Design review of the part built by this model. Coordinates are the model's own, in mm. A direction names the side the tool comes from. Coordinates: 2 decimals unless noted, no trailing zeros. Loops run counter-clockwise (first coordinate to the right, second up) from the corner with the lowest first, then second, coordinate; pieces in that order, holes last. Notation, with made-up numbers: (-19.75, -27) -> (36.25, -27) arc R25 cw to (36.25, 5) -> close; hole circle Ø8 at (-35.5, 86.25). An arc over 180 degrees is marked (long way). Use CSV: the item, a comma, the result in double quotes.
```python
from build123d import *

# Parameters (mm, degrees)
AUFSATZ_LINEAR_AUSTRAGEN1_DEPTH        = 6
F_3_5_3_5_DURCHMESSER_BOHRUNG1_D       = 3.5
F_3_0_3_DURCHMESSER_BOHRUNG2_OUTLINE_R = 1.5
F_3_0_3_DURCHMESSER_BOHRUNG2_DEPTH     = 6
SKIZZE10_R                             = 2.5
AUFSATZ_LINEAR_AUSTRAGEN2_DEPTH        = 4


# Read off the part's stored shape, not the designer's step: Ø3.0 (3) Durchmesser Bohrung2
with BuildPart() as part:
    # Skizze1 → Aufsatz-Linear austragen1 (new body)
    with BuildSketch(Plane.XY):
        with BuildLine():
            Line((-551.752498469, 213.343199998), (-551.752498469, 212.343199998))
            Line((-551.752498469, 212.343199998), (-555.752498469, 212.343199998))
            ThreePointArc((-555.752498469, 212.343199998), (-559.752498469, 208.343199998), (-555.752498469, 204.343199998))
            Line((-555.752498469, 204.343199998), (-551.752498469, 204.343199998))
            Line((-551.752498469, 204.343199998), (-551.752498469, 196.343199998))
            Line((-551.752498469, 196.343199998), (-555.752498469, 196.343199998))
            ThreePointArc((-555.752498469, 196.343199998), (-559.752498469, 192.343199998), (-555.752498469, 188.343199998))
            Line((-555.752498469, 188.343199998), (-551.752498469, 188.343199998))
            Line((-551.752498469, 188.343199998), (-551.752498469, 187.343199998))
            Line((-551.752498469, 187.343199998), (-532.752498469, 187.343199998))
            Line((-532.752498469, 187.343199998), (-532.752498469, 193.634996066))
            Line((-532.752498469, 193.634996066), (-519.752498469, 193.634996066))
            Line((-519.752498469, 193.634996066), (-519.752498469, 187.343199998))
            Line((-519.752498469, 187.343199998), (-500.752498469, 187.343199998))
            Line((-500.752498469, 187.343199998), (-500.752498469, 188.343199998))
            Line((-500.752498469, 188.343199998), (-496.752498469, 188.343199998))
            ThreePointArc((-496.752498469, 188.343199998), (-492.752498469, 192.343199998), (-496.752498469, 196.343199998))
            Line((-496.752498469, 196.343199998), (-500.752498469, 196.343199998))
            Line((-500.752498469, 196.343199998), (-500.752498469, 204.343199998))
            Line((-500.752498469, 204.343199998), (-496.752498469, 204.343199998))
            ThreePointArc((-496.752498469, 204.343199998), (-492.752498469, 208.343199998), (-496.752498469, 212.343199998))
            Line((-496.752498469, 212.343199998), (-500.752498469, 212.343199998))
            Line((-500.752498469, 212.343199998), (-500.752498469, 213.343199998))
            Line((-500.752498469, 213.343199998), (-551.752498469, 213.343199998))
        make_face()
    extrude(amount=AUFSATZ_LINEAR_AUSTRAGEN1_DEPTH)

    # Ø3.5 (3.5) Durchmesser Bohrung1 (through all)
    with Locations(Plane.XY.offset(6)):
        with Locations((-555.752498469, 208.343199998), (-555.752498469, 192.343199998), (-496.752498469, 192.343199998), (-496.752498469, 208.343199998)):
            Hole(F_3_5_3_5_DURCHMESSER_BOHRUNG1_D / 2)

    # Ø3.0 (3) Durchmesser Bohrung2 outline → Ø3.0 (3) Durchmesser Bohrung2 (cut)
    with BuildSketch(Plane.XY):
        with Locations((-546.902498469, 208.493199998)):
            Circle(F_3_0_3_DURCHMESSER_BOHRUNG2_OUTLINE_R)
        with Locations((-505.602498469, 192.193199998)):
            Circle(F_3_0_3_DURCHMESSER_BOHRUNG2_OUTLINE_R)
        with Locations((-546.902498469, 192.193199998)):
            Circle(F_3_0_3_DURCHMESSER_BOHRUNG2_OUTLINE_R)
        with Locations((-505.602498469, 208.493199998)):
            Circle(F_3_0_3_DURCHMESSER_BOHRUNG2_OUTLINE_R)
    extrude(amount=F_3_0_3_DURCHMESSER_BOHRUNG2_DEPTH, mode=Mode.SUBTRACT)

    # Skizze10 → Aufsatz-Linear austragen2 (add)
    with BuildSketch(Plane.XY.offset(6)):
        with Locations((-546.902498469, 208.493199998)):
            Circle(SKIZZE10_R)
        with Locations((-546.902498469, 192.193199998)):
            Circle(SKIZZE10_R)
        with Locations((-505.602498469, 208.493199998)):
            Circle(SKIZZE10_R)
        with Locations((-505.602498469, 192.193199998)):
            Circle(SKIZZE10_R)
    extrude(amount=AUFSATZ_LINEAR_AUSTRAGEN2_DEPTH)


solid = part.part
```
Item 1: Add section D-D (z = 8.75). Give the boundary of the cut face in (x, y).
Checked values:
outline,"circle Ø5 at (-546.9, 192.19); circle Ø5 at (-546.9, 208.49); circle Ø5 at (-505.6, 192.19); circle Ø5 at (-505.6, 208.49)"
Item 2: Add section C-C (y = 202.75). Give the boundary of the cut face in (x, z).
Checked values:
outline,"(-551.75, 0) -> (-500.75, 0) -> (-500.75, 6) -> (-551.75, 6) -> close"
Item 3: Machinability: for faces 1 (the face through (-554, 204.343, 3)), 2 (the face through (-504.91, 190.862, 2.958)), 3 (the face through (-500.752, 200, 3)), which of the approach directions +Z, -Z, +X, -X, +Y, -Y give a long, thin tool a straight path to every point of the face, cutting with its end or side? Answer none if there is none.
Checked values:
face 1,"+Z, -Z, -X"
face 2,"-Z"
face 3,"+Z, -Z, +X"
Item 4: Draft analysis for pull direction X (two halves, no side actions). For faces 4 (the face through (-506, 192, 6)), 5 (the face through (-549.4, 192.3, 8)), 6 (the face through (-554, 188.343, 3)), 7 (the face through (-559.75, 208.43, 2.96)), state which applies: pulls with the +X half, pulls with the -X half, needs draft (parallel to the pull), parting line crosses it, or undercut.
Checked values:
face 4,"undercut"
face 5,"undercut"
face 6,"needs draft"
face 7,"pulls with the -X half"
Item 5: Add section A-A (x = -505.5). Give the boundary of the cut face in (y, z).
Checked values:
outline,"(187.34, 0) -> (190.7, 0) -> (190.7, 6) -> (193.69, 6) -> (193.69, 0) -> (207, 0) -> (207, 6) -> (209.99, 6) -> (209.99, 0) -> (213.34, 0) -> (213.34, 6) -> (210.99, 6) -> (210.99, 10) -> (206, 10) -> (206, 6) -> (194.69, 6) -> (194.69, 10) -> (189.7, 10) -> (189.7, 6) -> (187.34, 6) -> close"
Item 6: Clearance check with flat-ended pins moving along their axes: pin 1 (5 mm diameter, centred on x = -550, z = 9, fed in from +Y); pin 2 (2 mm diameter, centred on x = -541.5, y = 199, fed in from +Z); pin 3 (0.5 mm diameter, centred on y = 187.5, z = 1.5, fed in from +X); pin 4 (3.5 mm diameter, centred on x = -546.5, y = 191.5, fed in from -Z). State where each tip first meets the part, or that it passes through.
Checked values:
pin 1,"y = 210.92"
pin 2,"z = 6"
pin 3,"x = -500.75"
pin 4,"z = 0"
Item 7: Add section B-B (z = 1.75). State how many separate pieces and enclosed holes the cut face has, then the cut area to 3 significant figures.
Checked values:
separate pieces,"1"
enclosed holes,"8"
area,"1,410 mm^2"
Item 8: To check wall thickness, follow line 1 along Y through (x, z) = (-506, 3.5); line 2 along X through (y, z) = (207.25, 9); line 3 along Z through (x, y) = (-533.5, 200). State the ranges of each line that lie inside material, in increasing order.
Checked values:
line 1,"187.34 to 190.75, 193.64 to 207.05, 209.94 to 213.34"
line 2,"-549.07 to -544.73, -507.77 to -503.43"
line 3,"0 to 6"
